from build123d import *

# Parameters (mm, degrees)
EXTRUDE_1_DEPTH = 2
EXTRUDE_2_DEPTH = 3.5
EXTRUDE_3_DEPTH = 4.55
FILLET_1_R      = 2
CHAMFER_1_SIZE  = 2
CHAMFER_2_SIZE  = 2


with BuildPart() as part:
    # Эскиз1 → Бобышка-Вытянуть1 (new body)
    with BuildSketch(Plane.XY):
        Polygon((46.296875, 9.92578125), (37.5703125, 13.70078125), (-18.703125, 13.70078125), (-18.703125, -11.29921875), (37.5703125, -11.29921875), (46.296875, -7.52421875), align=None)
    extrude(amount=EXTRUDE_1_DEPTH)

    # Эскиз2 → Бобышка-Вытянуть2 (add)
    with BuildSketch(Plane.XY.offset(2)):
        Polygon((-18.703125, -11.29921875), (37.5703125, -11.29921875), (46.296875, -7.52421875), (46.296875, 9.92578125), (37.5703125, 13.70078125), (-18.703125, 13.70078125), align=None)
        Polygon((-16.703125, 11.70078125), (33.296875, 11.70078125), (33.296875, 7.30078125), (43.596875, 7.30078125), (43.596875, -4.89921875), (33.296875, -4.89921875), (33.296875, -9.29921875), (-16.703125, -9.29921875), align=None, mode=Mode.SUBTRACT)
    extrude(amount=EXTRUDE_2_DEPTH)

    # Эскиз3 → Бобышка-Вытянуть3 (add)
    with BuildSketch(Plane.XY.offset(5.5)):
        Polygon((-18.703125, 13.70078125), (-18.703125, -11.29921875), (37.5703125, -11.29921875), (46.296875, -7.52421875), (46.296875, -4.89921875), (33.296875, -4.89921875), (33.296875, -9.29921875), (-16.703125, -9.29921875), (-16.703125, 11.70078125), (33.296875, 11.70078125), (33.296875, 7.30078125), (46.296875, 7.30078125), (46.296875, 9.92578125), (37.5703125, 13.70078125), align=None)
    extrude(amount=EXTRUDE_3_DEPTH)

    # Скругление1
    fillet_1_edges = [part.edges().sort_by_distance(p)[0] for p in [
        (-18.703125, 13.70078125, 5.025),
        (-18.703125, -11.29921875, 5.025),
    ]]
    fillet(fillet_1_edges, radius=FILLET_1_R)

    # Фаска1
    chamfer_1_edges = [part.edges().sort_by_distance(p)[0] for p in [
        (10.43359375, 13.70078125, 0),
        (10.43359375, -11.29921875, 0),
        (-18.703125, 1.20078125, 0),
        (-18.117338562, 13.114994812, 0),
        (-18.117338562, -10.713432312, 0),
    ]]
    chamfer(chamfer_1_edges, length=CHAMFER_1_SIZE)

    # Фаска2
    chamfer_2_edges = [part.edges().sort_by_distance(p)[0] for p in [
        (44.245265935, 10.81328125, 0),
        (46.296875, 1.20078125, 0),
        (44.245265935, -8.41171875, 0),
    ]]
    chamfer(chamfer_2_edges, length=CHAMFER_2_SIZE)


solid = part.part
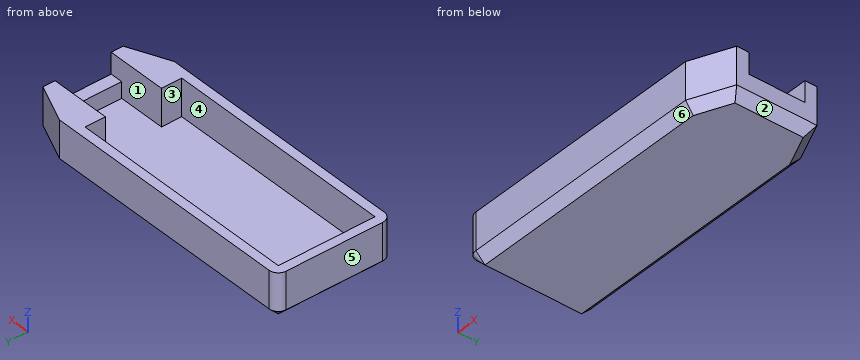
Check sheet for the modelled part. Datum: model origin and axes. Units: mm. Face numbers are marked on the shaded views. A direction names the side the tool comes from. Round coordinates to 2 decimals unless told otherwise and drop trailing zeros. Order: outer loops, then holes, each group sorted by start corner. A loop starts at its lowest first (then second) coordinate and runs counter-clockwise, first axis right, second up.
(1) Go/stop test with flat-tipped pins: P1, Ø3, axis at x = 45, y = 1, coming from the +Z side; P2, Ø1, axis at x = 25.5, y = 0.5, coming from the +Z side; P3, Ø2, axis at y = 5, z = 8, coming from the +X side. Record where each tip stops, or that it passes through.
(2) Cross-section at A-A, the plane z = 6.25. Enter the section's corners in (x, y).
(3) Cross-section at B-B, the plane x = 29. Enter the section's corners in (y, z), and give its area (3 significant figures).
(4) Access from +Z, -Z, +X, -X, +Y, -Y to the whole of each face (thin tool, end or side, straight path). Record for the marked faces 1 and 2.
(5) Cross-section at C-C, the plane z = 3. Enter the section's corners in (x, y).
(6) Cross-section at D-D, the plane y = -1. Enter the section's corners in (x, z), and give its area (3 significant figures).
(7) Draft check along Y on the marked faces 3, 4, 5 and 6. Enter one of: pulls with the +Y half, pulls with the -Y half, needs draft (parallel to the pull), parting line crosses it, or undercut.
(8) Scan lines: probe 1 along Y at (x, z) = (-4, 6.75); probe 2 along Y at (x, z) = (35, 6.5); probe 3 along X at (y, z) = (-5, 2.5). Record each from-to range of solid material in increasing order.
Check sheet entries:
1. P1: stops at z = 5.5
1. P2: stops at z = 2
1. P3: stops at x = -16.7
2. outline: (-18.7, -9.3) arc R2 ccw to (-16.7, -11.3) - (37.57, -11.3) - (46.3, -7.52) - (46.3, -4.9) - (33.3, -4.9) - (33.3, -9.3) - (-16.7, -9.3) - (-16.7, 11.7) - (33.3, 11.7) - (33.3, 7.3) - (46.3, 7.3) - (46.3, 9.93) - (37.57, 13.7) - (-16.7, 13.7) arc R2 ccw to (-18.7, 11.7) - close
3. outline: (-11.3, 2) - (-9.3, 0) - (11.7, 0) - (13.7, 2) - (13.7, 10.05) - (11.7, 10.05) - (11.7, 2) - (-9.3, 2) - (-9.3, 10.05) - (-11.3, 10.05) - close
3. area: 78.2 mm2
4. face 1: +Z
4. face 2: -Z, +X, +Y, -Y
5. outline: (-18.7, -9.3) arc R2 ccw to (-16.7, -11.3) - (37.57, -11.3) - (46.3, -7.52) - (46.3, 9.93) - (37.57, 13.7) - (-16.7, 13.7) arc R2 ccw to (-18.7, 11.7) - close; hole (-16.7, -9.3) - (33.3, -9.3) - (33.3, -4.9) - (43.6, -4.9) - (43.6, 7.3) - (33.3, 7.3) - (33.3, 11.7) - (-16.7, 11.7) - close
6. outline: (-18.7, 2) - (-16.7, 0) - (44.3, 0) - (46.3, 2) - (46.3, 5.5) - (43.6, 5.5) - (43.6, 2) - (-16.7, 2) - (-16.7, 10.05) - (-18.7, 10.05) - close
6. area: 152 mm2
7. face 3: undercut
7. face 4: undercut
7. face 5: needs draft
7. face 6: pulls with the -Y half
8. probe 1: y = -11.3 to -9.3, 11.7 to 13.7
8. probe 2: y = -11.3 to -4.9, 7.3 to 13.7
8. probe 3: x = -18.7 to -16.7, 33.3 to 46.3
